Part model, mm, in its own coordinate system. Face numbers are marked on the shaded views. A direction names the side the tool comes from. Coordinates: 2 decimals unless noted, no trailing zeros. Order: outer loops, then holes, each group sorted by start corner. A loop starts at its lowest first (then second) coordinate and runs counter-clockwise, first axis right, second up.
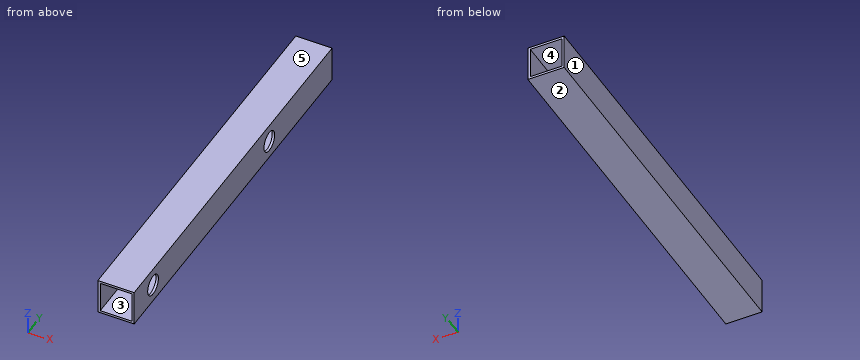
Autodesk Inventor part; units mm, degrees
ref_plane "YZ Plane" through (0, 0, 0) normal (1, 0, 0) x (0, 1, 0)
ref_plane "XZ Plane" through (0, 0, 0) normal (0, 1, 0) x (-1, 0, 0)
ref_plane "XY Plane" through (0, 0, 0) normal (0, 0, 1) x (1, 0, 0)
sketch "Sketch9" plane through (0, 0, 0) normal (0, 1, 0) x (-1, 0, 0)
  line L0 (15, 15) -> (-15, 15)
  line L1 (-15, 15) -> (-15, -15)
  line L2 (-15, -15) -> (15, -15)
  line L3 (15, -15) -> (15, 15)
  line L4 (15, 15) -> (-15, -15) construction
  line L5 (-15, 15) -> (15, -15) construction
  line L6 (-13, 13) -> (13, 13)
  line L7 (13, 13) -> (13, -13)
  line L8 (13, -13) -> (-13, -13)
  line L9 (-13, -13) -> (-13, 13)
  point P0 (0, 0)
  dimension "d172" = 30
  dimension "d173" = 30
  dimension "d174" = 2
extrude "Extrusion3" add sketch "Sketch9" against normal blind 315
sketch "Sketch10" plane through (0, 0, 0) normal (1, 0, 0) x (0, 1, 0)
  line L0 (0, 15) -> (0, -15) construction
  line L1 (0, 15) -> (-315, 15) construction
  line L2 (-315, -15) -> (-315, 15) construction
  line L3 (0, -15) -> (-315, -15) construction
  line L4 (-108.5, 8.5) -> (-91.5, 8.5)
  line L5 (-91.5, 8.5) -> (-91.5, -8.5)
  line L6 (-91.5, -8.5) -> (-108.5, -8.5)
  line L7 (-108.5, -8.5) -> (-108.5, 8.5)
  line L8 (-108.5, 8.5) -> (-91.5, -8.5) construction
  line L9 (-91.5, 8.5) -> (-108.5, -8.5) construction
  line L10 (-293.5, 8.5) -> (-276.5, 8.5)
  line L11 (-276.5, 8.5) -> (-276.5, -8.5)
  line L12 (-276.5, -8.5) -> (-293.5, -8.5)
  line L13 (-293.5, -8.5) -> (-293.5, 8.5)
  line L14 (-293.5, 8.5) -> (-276.5, -8.5) construction
  line L15 (-276.5, 8.5) -> (-293.5, -8.5) construction
  line L16 (-413.5, 8.5) -> (-396.5, 8.5)
  line L17 (-396.5, 8.5) -> (-396.5, -8.5)
  line L18 (-396.5, -8.5) -> (-413.5, -8.5)
  line L19 (-413.5, -8.5) -> (-413.5, 8.5)
  line L20 (-413.5, 8.5) -> (-396.5, -8.5) construction
  line L21 (-396.5, 8.5) -> (-413.5, -8.5) construction
  circle A0 centre (-470, 0) radius 8.5
  line L22 (0, 0) -> (30, 0)
  circle A1 centre (-100, 0) radius 8.5
  circle A2 centre (-285, 0) radius 8.5
  circle A3 centre (-405, 0) radius 8.5
  dimension "d177" = 17
  dimension "d178" = 17
  dimension "d181" = 30
  dimension "d182" = 130
  dimension "d183" = 315
  dimension "d184" = 435
  dimension "d185" = 500
  dimension "d186" = 17
extrude "Extrusion4" cut sketch "Sketch10" along normal through all contours A1 | A2
properties part number "SLM 1662 FDS 1000 way tube 2" material "Stainless Steel"
Q1. Which spindle directions (+Z, -Z, +X, -X, +Y, -Y) get a long thin tool onto all of the face, cutting with end or side? Do the marked faces 4 and 5. Say none if no direction does.
Results list:
face 4: +Y, -Y
face 5: +Z, +X, -X, +Y, -Y
Q2. Cut at A-A on x = 7.5. Write the cut outline in (y, z).
Results list:
outline: (-315, -15) - (0, -15) - (0, -13) - (-315, -13) - close; (-315, 13) - (0, 13) - (0, 15) - (-315, 15) - close
Q3. Cut at C-C on z = 0. Write the cut outline in (x, y).
Results list:
outline: (-15, -315) - (-13, -315) - (-13, 0) - (-15, 0) - close; (13, -315) - (15, -315) - (15, -293.5) - (13, -293.5) - close; (13, -276.5) - (15, -276.5) - (15, -108.5) - (13, -108.5) - close; (13, -91.5) - (15, -91.5) - (15, 0) - (13, 0) - close
Q4. Pin check, flat tip, straight feed: pin 1 Ø13.5 at (y, z) = (-285, 0) entering from +X. Stop position of the tip, or through.
Results list:
pin 1: stops at x = -13
Q5. Cut at D-D on y = -285. Write the cut outline in (x, z), and give its area (3 significant figures).
Results list:
outline: (-15, -15) - (15, -15) - (15, -8.5) - (13, -8.5) - (13, -13) - (-13, -13) - (-13, 13) - (13, 13) - (13, 8.5) - (15, 8.5) - (15, 15) - (-15, 15) - close
area: 190 mm2
Q6. Cut at B-B on y = -175. Write the cut outline in (x, z).
Results list:
outline: (-15, -15) - (15, -15) - (15, 15) - (-15, 15) - close; hole (-13, -13) - (13, -13) - (13, 13) - (-13, 13) - close
Q7. Wall check: line 1 along Y through (x, z) = (13.55, 0); line 2 along Z through (x, y) = (14.5, -100); line 3 along Z through (x, y) = (-10.75, -213.5). Give the ranges that are in metal, low to high.
Results list:
line 1: y = -315 to -293.5, -276.5 to -108.5, -91.5 to 0
line 2: z = -15 to -8.5, 8.5 to 15
line 3: z = -15 to -13, 13 to 15
Q8. Mould opens along Z. For the marked faces 1, 2 and 3 say: pulls with the +Z half, pulls with the -Z half, needs draft (parallel to the pull), parting line crosses it, or undercut.
Results list:
face 1: needs draft
face 2: pulls with the -Z half
face 3: undercut
